Can you work these out from the drawing? Everything is in mm from the part's minimum corner. A direction names the side the tool comes from. Round coordinates to 2 decimals unless told otherwise and drop trailing zeros. Loops run counter-clockwise (first coordinate to the right, second up) from the corner with the lowest first, then second, coordinate; pieces in that order, holes last. Notation, with made-up numbers: (67, 68) -> (103, 68) arc R12 ccw to (103, 72) -> close; hole circle Ø7 at (-6.5, 0). An arc over 180 degrees is marked (long way). One line per item, written item: value.
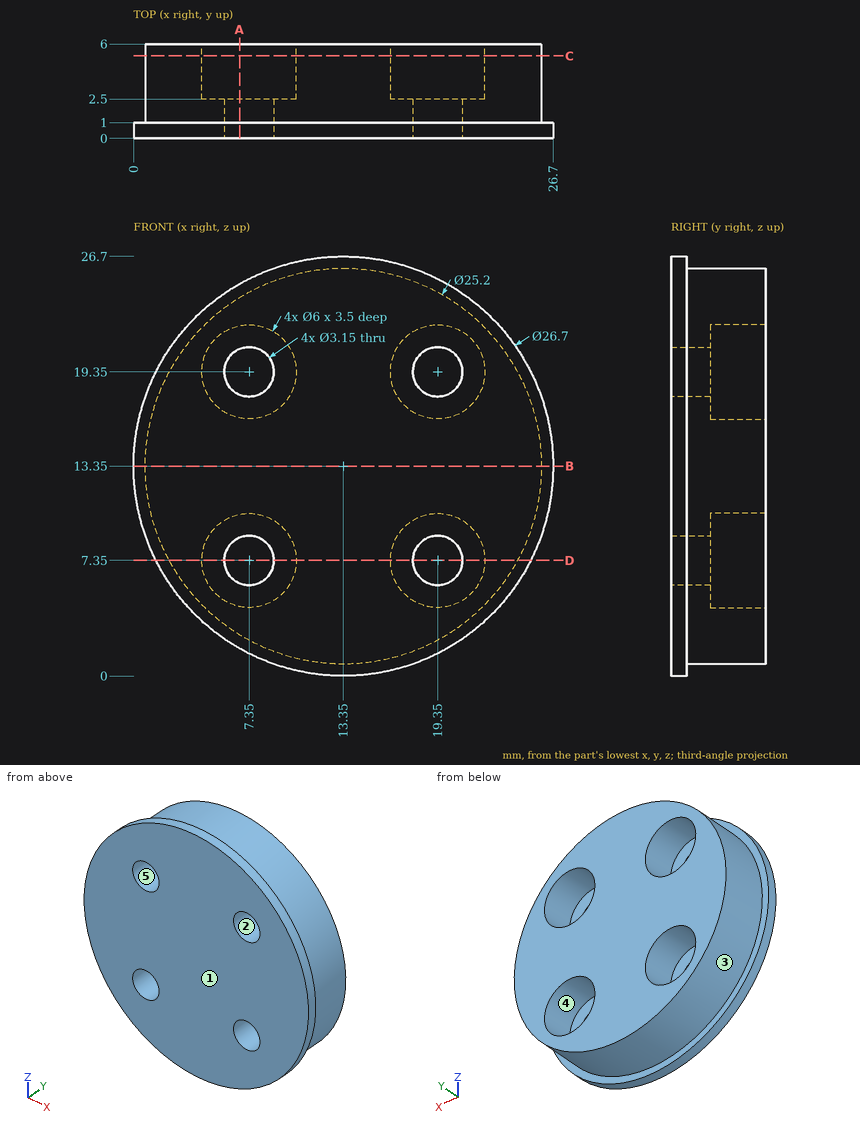
Item 1: I need wall thicknesses on line 1 (X direction, y = 0.75, z = 6); line 2 (Z direction, x = 7.35, y = 0.95) (3 decimals); line 3 (Z direction, x = 5.75, y = 5.1). Which ranges of each line are inside material? Lowest first, please. Write a range as from..to.
Output:
line 1: x = 2.21..6.54, 8.16..18.54, 20.16..24.49
line 2: z = 1.424..5.775, 8.925..17.775, 20.925..25.276
line 3: z = 3.3..4.81, 9.89..16.81, 21.89..23.4
Item 2: If we section it at C-C on y = 5.25: List the corners of the cut face in (x, z) for me, plus the area to 3 significant figures.
Output:
outline: circle Ø25.2 at (13.35, 13.35); hole circle Ø6 at (7.35, 7.35); hole circle Ø6 at (7.35, 19.35); hole circle Ø6 at (19.35, 7.35); hole circle Ø6 at (19.35, 19.35)
area: 386 mm²
Item 3: Will these pins go through, and if not, where does the flat tip stop? pin 1 Ø5 at (x, z) = (19, 8.5) entering from +Y; pin 2 Ø2 at (x, y) = (17, 1.5) entering from +Z; pin 3 Ø5 at (x, z) = (19.35, 7.35) entering from +Y; pin 4 Ø2 at (y, z) = (1.5, 3.5) entering from +X.
Output:
pin 1: stops at y = 6
pin 2: stops at z = 26.41
pin 3: stops at y = 2.5
pin 4: stops at x = 23.22
Item 4: If we section it at D-D on z = 7.35: List the corners of the cut face in (x, y) for me (3 decimals), plus the area to 3 significant figures.
Output:
outline: (1.424, 0) -> (5.775, 0) -> (5.775, 2.5) -> (4.35, 2.5) -> (4.35, 6) -> (2.27, 6) -> (2.27, 1) -> (1.424, 1) -> close; (8.925, 0) -> (17.775, 0) -> (17.775, 2.5) -> (16.35, 2.5) -> (16.35, 6) -> (10.35, 6) -> (10.35, 2.5) -> (8.925, 2.5) -> close; (20.925, 0) -> (25.276, 0) -> (25.276, 1) -> (24.43, 1) -> (24.43, 6) -> (22.35, 6) -> (22.35, 2.5) -> (20.925, 2.5) -> close
area: 76.9 mm²
Item 5: If we section it at B-B on z = 13.35: List the corners of the cut face in (x, y) for me, plus the area to 3 significant figures.
Output:
outline: (0, 0) -> (26.7, 0) -> (26.7, 1) -> (25.95, 1) -> (25.95, 6) -> (0.75, 6) -> (0.75, 1) -> (0, 1) -> close
area: 153 mm²
Item 6: If we mould it in two halves opening along X, with no side actions, what happens to the marked faces 1, 2 and 3? For each: released by +X, released by -X, zero draft, split by the parting line, or undercut.
Output:
face 1: zero draft
face 2: undercut
face 3: split by the parting line
Item 7: If we section it at A-A on x = 6.75: List the corners of the cut face in (y, z) for me, plus the area to 3 significant figures.
Output:
outline: (0, 1.75) -> (1, 1.75) -> (1, 2.62) -> (6, 2.62) -> (6, 4.41) -> (2.5, 4.41) -> (2.5, 5.89) -> (0, 5.89) -> close; (0, 8.81) -> (2.5, 8.81) -> (2.5, 10.29) -> (6, 10.29) -> (6, 16.41) -> (2.5, 16.41) -> (2.5, 17.89) -> (0, 17.89) -> close; (0, 20.81) -> (2.5, 20.81) -> (2.5, 22.29) -> (6, 22.29) -> (6, 24.08) -> (1, 24.08) -> (1, 24.95) -> (0, 24.95) -> close
area: 74.8 mm²
Item 8: For the marked faces 4 and 5, which set-ups out of +Z, -Z, +X, -X, +Y, -Y let a thin tool reach every point of the face, with its end or its side?
Output:
face 4: +Y
face 5: +Y, -Y
